Build history of the part. All positions in model axes, mm. Face numbers are marked on the shaded views. Give positions to 0.01 mm unless a question says otherwise; leave off trailing zeros. Order: outer loops, then holes, each group sorted by start corner. A loop starts at its lowest first (then second) coordinate and runs counter-clockwise, first axis right, second up. Notation, with made-up numbers: (56.25, 47) - (111.25, 47) arc R23 cw to (111.25, 85) - close; hole circle Ø10 at (-8, -5.75). An arc over 180 degrees is marked (long way). Use a Markdown table: item, result. Add a question column.
(1) Slice it at C-C (x = -262.5). Write the cut outline in (y, z).
(2) Slice it at A-A (z = 48). Write the cut outline in (x, y) (3 decimals), then the cut area to 3 significant figures.
(3) Slice it at B-B (y = 23.5). Write the cut outline in (x, z) (3 decimals).
(4) Mould opens along X. For the marked faces 1, 2, 3 and 4 say: +X half, -X half, draft (parallel to the pull), parting line (faces both ways), or undercut.
(5) Wall check: line 1 (Y direction, x = 118, z = 29.5); line 2 (X direction, y = -12, z = 73.5) (3 decimals); line 3 (Z direction, x = -34, y = -17.5). Give the ranges that are in metal, low to high.
(6) Flat gauge pins, fed straight in: pin 1 (20 mm diameter, centred on x = 282, y = -50, fed in from +Z); pin 2 (9 mm diameter, centred on x = -87, y = -44, fed in from +Z); pin 3 (12 mm diameter, centred on x = -173, z = 27.5, fed in from -Y). Where does each tip first touch, or does it go through?
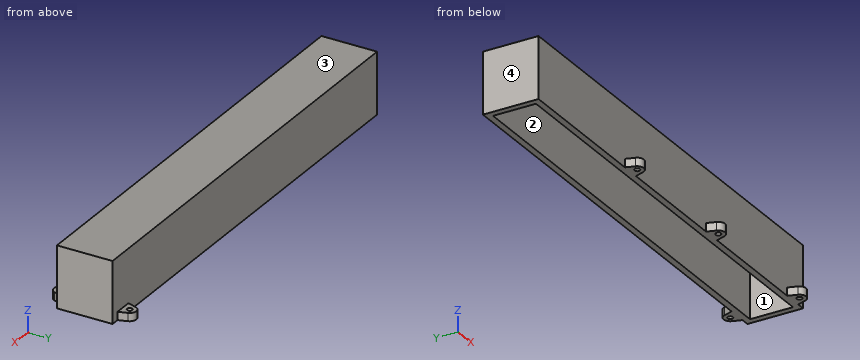
from build123d import *

# Parameters (mm, degrees)
F0_W     = 603.25
F0_H     = 75.6
F1_DEPTH = 83.4
F2_T     = -8.6
F4_START = -72.4
F3_R     = 3.6
F4_DEPTH = 11
F5_R     = 3.6
F6_DEPTH = 11.3


with BuildPart() as f1:
    # F0 (on Top) → F1 (new body)
    with BuildSketch(Plane.XY):
        Rectangle(F0_W, F0_H)
    extrude(amount=F1_DEPTH)

    # F2
    f2_openings = [f1.faces().sort_by_distance(p)[0] for p in [
        (0, 0, 0),
    ]]
    offset(amount=F2_T, openings=f2_openings)

    # F3 (on face) → F4 (join)
    with BuildSketch(Plane.XY.offset(83.4).offset(F4_START)):
        with BuildLine():
            Line((290.425, 37.8), (286.3608661331, 49.8865758556))
            ThreePointArc((286.3608661331, 49.8865758556), (277.925, 55.95), (269.4891338669, 49.8865758556))
            Line((269.4891338669, 49.8865758556), (265.425, 37.8))
            Line((265.425, 37.8), (290.425, 37.8))
        make_face()
        with Locations((277.925, 47.05)):
            Circle(F3_R, mode=Mode.SUBTRACT)
        with BuildLine():
            Line((290.425, -37.8), (265.425, -37.8))
            Line((265.425, -37.8), (269.4891338669, -49.8865758556))
            ThreePointArc((269.4891338669, -49.8865758556), (277.925, -55.95), (286.3608661331, -49.8865758556))
            Line((286.3608661331, -49.8865758556), (290.425, -37.8))
        make_face()
        with Locations((277.925, -47.05)):
            Circle(F3_R, mode=Mode.SUBTRACT)
    extrude(amount=-F4_DEPTH)

    # F5 (on face) → F6 (join)
    with BuildSketch(Plane(origin=(0, 0, 0), x_dir=(1, 0, 0), z_dir=(0, 0, -1))):
        with BuildLine():
            Line((80.425, 37.8), (105.425, 37.8))
            Line((105.425, 37.8), (101.3608661331, 49.8865758556))
            ThreePointArc((101.3608661331, 49.8865758556), (92.925, 55.95), (84.4891338669, 49.8865758556))
            Line((84.4891338669, 49.8865758556), (80.425, 37.8))
        make_face()
        with Locations((92.925, 47.05)):
            Circle(F5_R, mode=Mode.SUBTRACT)
        with BuildLine():
            Line((-104.575, 37.8), (-79.575, 37.8))
            Line((-79.575, 37.8), (-83.6391338669, 49.8865758556))
            ThreePointArc((-83.6391338669, 49.8865758556), (-92.075, 55.95), (-100.5108661331, 49.8865758556))
            Line((-100.5108661331, 49.8865758556), (-104.575, 37.8))
        make_face()
        with Locations((-92.075, 47.05)):
            Circle(F5_R, mode=Mode.SUBTRACT)
    extrude(amount=-F6_DEPTH)


solid = f1.part
Solution:
| question | item | result |
|---|---|---|
| 1 | outline | (-37.8, 0) - (-29.2, 0) - (-29.2, 74.8) - (29.2, 74.8) - (29.2, 0) - (37.8, 0) - (37.8, 83.4) - (-37.8, 83.4) - close |
| 2 | outline | (-301.625, -37.8) - (301.625, -37.8) - (301.625, 37.8) - (-301.625, 37.8) - close; hole (-293.025, -29.2) - (293.025, -29.2) - (293.025, 29.2) - (-293.025, 29.2) - close |
| 2 | area | 11,400 mm2 |
| 3 | outline | (-301.625, 0) - (-293.025, 0) - (-293.025, 74.8) - (293.025, 74.8) - (293.025, 0) - (301.625, 0) - (301.625, 83.4) - (-301.625, 83.4) - close |
| 4 | face 1 | undercut |
| 4 | face 2 | undercut |
| 4 | face 3 | draft |
| 4 | face 4 | -X half |
| 5 | line 1 | -37.8 to -29.2, 29.2 to 37.8 |
| 5 | line 2 | -301.625 to -293.025, 293.025 to 301.625 |
| 5 | line 3 | 74.8 to 83.4 |
| 6 | pin 1 | z = 11 |
| 6 | pin 2 | z = 11.3 |
| 6 | pin 3 | y = -37.8 |
